Autodesk Inventor part; units mm, degrees
ref_plane "YZ Plane" through (0, 0, 0) normal (1, 0, 0) x (0, 1, 0)
ref_plane "XZ Plane" through (0, 0, 0) normal (0, 1, 0) x (-1, 0, 0)
ref_plane "XY Plane" through (0, 0, 0) normal (0, 0, 1) x (1, 0, 0)
sketch "Sketch1" plane through (0, 0, 0) normal (0, 0, 1) x (1, 0, 0)
  line L0 (14.8889, 11.5915) -> (26.8889, 11.5915)
  line L1 (26.8889, 11.5915) -> (26.8889, -6.9085)
  line L2 (26.8889, -6.9085) -> (14.8889, -6.9085)
  line L3 (14.8889, -6.9085) -> (14.8889, 11.5915)
  line L4 (14.8889, 11.5915) -> (-10.1111, 11.5915)
  line L5 (-10.1111, 11.5915) -> (-10.1111, 7.5915)
  line L6 (-10.1111, 7.5915) -> (14.8889, 7.5915)
  line L7 (14.8889, 7.5915) -> (14.8889, 11.5915)
  line L8 (14.8889, -6.9085) -> (-10.1111, -6.9085)
  line L9 (-10.1111, -6.9085) -> (-10.1111, -2.9085)
  line L10 (-10.1111, -2.9085) -> (14.8889, -2.9085)
  line L11 (14.8889, -2.9085) -> (14.8889, -6.9085)
  point P0 (0, 0)
  dimension "d0" = 10.5
  dimension "d1" = 4
  dimension "d2" = 4
  dimension "d3" = 12
  dimension "d4" = 25
extrude "Extrusion1" add sketch "Sketch1" along normal blind 30
sketch "Sketch2" plane through (-10.1111, -6.9085, 0) normal (0, -1, 0) x (1, 0, 0)
  line L0 (0, 30) -> (37, 30)
  line L1 (0, 0) -> (37, 0)
  line L2 (25, 0) -> (25, 30)
  point P0 (10.1111, 0)
  point P1 (18, 25)
  point P2 (18, 5)
  point P3 (8, 5)
  dimension "d7" = 5
  dimension "d8" = 5
  dimension "d9" = 5
  dimension "d10" = 10
  dimension "d11" = 0
  dimension "d12" = 7
hole "Hole1" at (7.8889, -6.9085, 25) at (7.8889, -6.9085, 5) at (-2.1111, -6.9085, 5) direction (0, 1, 0) diameter 3 depth 8 tip angle 118 countersink diameter 6 countersink angle 90
sketch "Sketch3" plane through (-10.1111, 11.5915, 0) normal (0, 1, 0) x (1, 0, 0)
  circle A0 centre (18, -25) radius 1.5
  circle A1 centre (18, -5) radius 1.5
  circle A2 centre (8, -5) radius 1.5
  point P0 (10.1111, 0)
hole "Hole2" at (7.8889, 11.5915, 25) at (7.8889, 11.5915, 5) at (-2.1111, 11.5915, 5) direction (0, -1, 0) diameter 3 depth 8 tip angle 118 counterbore diameter 6 counterbore depth 2
chamfer "Chamfer1" distance 5 angle 45 1 edges at (26.8889, 2.3415, 0)
sketch "Sketch4" plane through (0, 0, 30) normal (0, 0, 1) x (1, 0, 0)
  line L0 (21.8889, 11.5915) -> (14.8889, 11.5915)
  line L1 (14.8889, 11.5915) -> (14.8889, 71.5915)
  line L2 (14.8889, 71.5915) -> (21.8889, 71.5915)
  line L3 (21.8889, 71.5915) -> (21.8889, 11.5915)
  line L4 (-10.1111, -6.9085) -> (21.8889, -6.9085)
  line L5 (14.8889, -6.9085) -> (21.8889, -6.9085)
  line L6 (21.8889, -6.9085) -> (21.8889, -66.9085)
  line L7 (21.8889, -66.9085) -> (14.8889, -66.9085)
  line L8 (14.8889, -66.9085) -> (14.8889, -6.9085)
  line L9 (14.8889, 7.5915) -> (14.8889, -2.9085)
  point P0 (0, 0)
  dimension "d30" = 60
  dimension "d31" = 60
extrude "Extrusion2" add sketch "Sketch4" against normal blind 30
sketch "Sketch5" plane through (0, 0, 30) normal (0, 0, 1) x (1, 0, 0)
  line L0 (14.8889, 7.5915) -> (14.8889, -2.9085)
  line L1 (14.8889, 2.3415) -> (26.8889, 2.3415)
  line L2 (26.8889, 2.3415) -> (26.8889, 27.3415)
  line L3 (26.8889, 27.3415) -> (14.8889, 27.3415)
  line L4 (14.8889, 27.3415) -> (14.8889, 2.3415)
  line L5 (14.8889, 2.3415) -> (26.8889, 2.3415)
  line L6 (26.8889, 2.3415) -> (26.8889, -22.6585)
  line L7 (26.8889, -22.6585) -> (14.8889, -22.6585)
  line L8 (14.8889, -22.6585) -> (14.8889, 2.3415)
  line L9 (26.8889, -6.9085) -> (26.8889, 11.5915)
  point P0 (0, 0)
  dimension "d34" = 25
  dimension "d35" = 25
extrude "Extrusion3" add sketch "Sketch5" against normal blind 30
sketch "Sketch6" plane through (0, 0, 30) normal (0, 0, 1) x (1, 0, 0)
  line L0 (26.8889, -22.6585) -> (26.8889, 27.3415)
  line L1 (26.8889, 27.3415) -> (21.8889, 27.3415)
  circle A0 centre (20.8889, 22.3415) radius 3.5
  circle A1 centre (20.8889, -17.6585) radius 3.5
  point P0 (0, 0)
  dimension "d38" = 40
  dimension "d39" = 6
  dimension "d40" = 6
  dimension "d41" = 5
  dimension "d42" = 7
  dimension "d43" = 7
extrude "Extrusion4" cut sketch "Sketch6" against normal blind 20
chamfer "Chamfer2" distance 5 angle 45 2 edges at (21.8889, -22.6585, 15) (21.8889, 27.3415, 15)
chamfer "Chamfer3" distance 20 distance2 40 1 edges at (18.3889, -66.9085, 30) measured on face at (19.5556, -66.9085, 20)
chamfer "Chamfer4" distance 20 distance2 40 1 edges at (18.3889, 71.5915, 30) measured on face at (17.2222, 71.5915, 20)
sketch "Sketch7" plane through (26.8889, -22.6585, 30) normal (1, 0, 0) x (0, 0, -1)
  point P0 (30, 22.6585)
sketch "Sketch8" plane through (14.8889, -66.9085, 0) normal (-1, 0, 0) x (0, 0, 1)
  line L0 (0, 94.25) -> (0, 44.25)
  line L1 (0, 74.5) -> (0, 64)
  point P0 (0, 66.9085)
  point P1 (5, 84.25)
  point P2 (5, 54.25)
  point P3 (0, 69.25)
  dimension "d55" = 30
  dimension "d56" = 5
  dimension "d57" = 5
  dimension "d58" = 15
hole "Hole3" at (14.8889, -12.6585, 5) at (14.8889, 17.3415, 5) direction (1, 0, 0) diameter 3 depth 20 tip angle 118 countersink diameter 6 countersink angle 90
sketch "Sketch9" plane through (14.8889, 11.5915, 0) normal (-1, 0, 0) x (0, 0, 1)
  point P0 (0, -11.5915)
sketch "Sketch10" plane through (26.8889, -22.6585, 30) normal (1, 0, 0) x (0, 0, -1)
  line L0 (0, 30.25) -> (0, 19.75)
  point P0 (30, 22.6585)
  point P1 (5, 25)
  dimension "d66" = 5
hole "Hole4" at (26.8889, 2.3415, 25) direction (-1, 0, 0) diameter 3 depth 20 tip angle 118
properties part number "Col support beam"
Can you work these out from the model? Positions are in its coordinate system, mm. A direction names the side the tool comes from. Coordinates: 2 decimals unless noted, no trailing zeros. Loops run counter-clockwise (first coordinate to the right, second up) from the corner with the lowest first, then second, coordinate; pieces in that order, holes last.
1) Imagine slicing it at A-A on z = 18. State how many separate pieces and enclosed holes the cut face has, plus the area to 3 significant figures.
2) For pin 1 (5 mm diameter, centred on x = 7.89, z = 25, fed in from -Y); pin 2 (1 mm diameter, centred on x = -5.5, z = 11, fed in from -Y); pin 3 (8 mm diameter, centred on x = 7.89, z = 25, fed in from +Y), each with a flat end and sliding along its axis, tell me the tip position at first contact or that it passes through.
3) Which directions (+Z, -Z, +X, -X, +Y, -Y) give clear straight access to the entire face, cutting with the end or side of a thin tool? Please do faces 1 (the cylindrical face through (22.77, 25.293, 20.14)), 2 (the flat face through (-0.8, 9.592, 6.3)), 3 (the flat face through (14.889, 2, 15)).
4) I need wall thicknesses on probe 1 along X at (y, z) = (10, 5); probe 2 along X at (y, z) = (-4.7, 5); probe 3 along Y at (x, z) = (1.5, 9.5). Which ranges of each line are inside material? Lowest first, please.
5) Thinking about a two-plate mould opening in Y: for faces 4 (the flat face through (17.85, 51.31, 20.14)), 5 (the flat face through (18, -66.908, 5)), 6 (the cylindrical face through (21.71, -13.92, 5.81)), which applies, pulls with the +Y half, pulls with the -Y half, needs draft (parallel to the pull), parting line crosses it, or undercut?
6) Imagine slicing it at D-D on y = -56. List the corners of the cut face in (x, z) for me.
Completed:
1. separate pieces: 1
1. enclosed holes: 2
1. area: 1,140 mm2
2. pin 1: stops at y = -6.41
2. pin 2: stops at y = -6.91
2. pin 3: stops at y = 11.59
3. face 1: +Z
3. face 2: +Y
3. face 3: +Z, -Z, -X
4. probe 1: x = -10.11 to -5.11, 0.89 to 4.89, 10.89 to 26.89
4. probe 2: x = -10.11 to -3.61, -0.61 to 6.39, 9.39 to 26.89
4. probe 3: y = -6.91 to -2.91, 7.59 to 11.59
5. face 4: pulls with the +Y half
5. face 5: pulls with the -Y half
5. face 6: undercut
6. outline: (14.89, 0) - (21.89, 0) - (21.89, 15.45) - (14.89, 15.45) - close
